Geometry check sheet. Reference: the model listing, model coordinates, mm. A direction names the side the tool comes from. Round coordinates to 2 decimals unless told otherwise and drop trailing zeros. Write each loop counter-clockwise with the first axis right and the second up, starting at its lowest first coordinate (ties: lowest second). Pieces come first, ordered by that corner, then holes. Notation, with made-up numbers: (-6, 37.5) - (31, 37.5) arc R20 cw to (31, 47.5) - close; hole circle Ø2 at (-27.5, 26). An arc over 180 degrees is marked (long way). Return JSON: item names as keys, results as strings.
Autodesk Inventor part; units mm, degrees
ref_plane "YZ Plane" through (0, 0, 0) normal (1, 0, 0) x (0, 1, 0)
ref_plane "XZ Plane" through (0, 0, 0) normal (0, 1, 0) x (-1, 0, 0)
ref_plane "XY Plane" through (0, 0, 0) normal (0, 0, 1) x (1, 0, 0)
sketch "スケッチ1" plane through (0, 0, 0) normal (1, 0, 0) x (0, 1, 0)
  circle A0 centre (0, 0) radius 19.6
  circle A1 centre (0, 19.6) radius 1.4
  circle A2 centre (-19.6, 0) radius 1.4
  circle A3 centre (0, -19.6) radius 1.4
  circle A4 centre (19.6, 0) radius 1.4
  circle A5 centre (0, 0) radius 50
  dimension "d0" = 39.2
  dimension "d1" = 2.8
  dimension "d4" = 360
  dimension "d6" = 100
extrude "押し出し1" add sketch "スケッチ1" along normal blind 2 contours A4 A0 A3 A2 A1 | A5
sketch "スケッチ2" plane through (0, 0, 0) normal (-1, 0, 0) x (0, 0, 1)
  circle A0 centre (0, 0) radius 50
  circle A1 centre (0, 0) radius 37.5
  dimension "d9" = 75
extrude "押し出し2" add sketch "スケッチ2" along normal blind 7
sketch "スケッチ3" plane through (2, 0, 0) normal (1, 0, 0) x (0, 0, -1)
  circle A0 centre (0, 0) radius 43.75
  circle A1 centre (-43.75, 0) radius 2.25
  circle A2 centre (43.75, 0) radius 2.25
  dimension "d12" = 87.5
  dimension "d13" = 4.5
  dimension "d14" = 4.5
extrude "押し出し3" cut sketch "スケッチ3" against normal blind 10 contours A0 A2 | A0 A2 | A1 A0 | A0 A1
sketch "スケッチ4" plane through (2, 0, 0) normal (1, 0, 0) x (0, 0, -1)
  circle A0 centre (-43.75, 0) radius 2.25
  circle A1 centre (-43.75, 0) radius 4
  circle A2 centre (43.75, 0) radius 2.25
  circle A3 centre (43.75, 0) radius 4
  point P0 (0, 0)
  dimension "d17" = 8
  dimension "d18" = 8
extrude "押し出し4" cut sketch "スケッチ4" against normal blind 5
properties part number "laboratory_equipment-GIM3505-8" material "ABS プラスチック"
(1) Section check D-D, the plane z = -36. Enter the section's corners in (x, y).
Response values:
{"outline": "(-7, -34.7) - (2, -34.7) - (2, 34.7) - (-7, 34.7) - (-7, 10.5) - (0, 10.5) - (0, -10.5) - (-7, -10.5) - close"}
(2) Gauge pin test, flat ends, axial feed: pin 1 (9 mm diameter, centred on y = 0.5, z = -44.5, fed in from +X); pin 2 (2.5 mm diameter, centred on y = 0, z = 45, fed in from +X); pin 3 (3.5 mm diameter, centred on y = 0, z = 19.6, fed in from -X); pin 4 (1.5 mm diameter, centred on x = -4, z = -31, fed in from +Y). Record the tip position at first contact, or that the pin passes through.
Response values:
{"pin 1": "stops at x = 2", "pin 2": "stops at x = -3", "pin 3": "stops at x = 0", "pin 4": "stops at y = 39.81"}
(3) Section check A-A, the plane y = -19.6. Enter the section's corners in (x, z).
Response values:
{"outline": "(-7, -46) - (2, -46) - (2, -1.4) - (0, -1.4) - (0, -31.97) - (-7, -31.97) - close; (-7, 31.97) - (0, 31.97) - (0, 1.4) - (2, 1.4) - (2, 46) - (-7, 46) - close"}
(4) Access from +Z, -Z, +X, -X, +Y, -Y to the whole of each face (thin tool, end or side, straight path). Record for faces 4 (the face through (-3.45, -37.18, -4.88)), 5 (the face through (-5, 0, 46)), 6 (the face through (-3, -1.7, -45.5)).
Response values:
{"face 4": "-X", "face 5": "+X, -X", "face 6": "+X"}
(5) Section check B-B, the plane x = -5.25. Enter the section's corners in (y, z).
Response values:
{"outline": "circle Ø100 at (0, 0); hole circle Ø75 at (0, 0); hole circle Ø4.5 at (0, -43.75); hole circle Ø4.5 at (0, 43.75)"}
(6) Release check for a two-part mould opening along Y. For faces 1 (the face through (2, -1, 1)), 2 (the face through (-3, -2, 42)), 3 (the face through (0.99, 0.75, -20.78)) record: pulls with the +Y half, pulls with the -Y half, needs draft (parallel to the pull), parting line crosses it, or undercut.
Response values:
{"face 1": "needs draft", "face 2": "undercut", "face 3": "undercut"}
(7) Material ranges on line 1 along X through (y, z) = (-12.5, 22.5); line 2 along Z through (x, y) = (0.6, 19.6); line 3 along Z through (x, y) = (-1.5, -10), recorded low to high. Write a range as [from, to].
Response values:
{"line 1": "x = [0, 2]", "line 2": "z = [-46, -1.4], [1.4, 46]", "line 3": "z = [-48.99, -36.14], [36.14, 48.99]"}
